```python
from build123d import *

# Parameters (mm, degrees)
SKETCH1_R           = 3.3782
SKETCH1_R_2         = 6
SKETCH1_R_3         = 8
BOSS_EXTRUDE1_DEPTH = 4.826
SKETCH2_W           = 4.826
SKETCH2_H           = 25.4
BOSS_EXTRUDE2_DEPTH = 4.826
SKETCH3_W           = 4.826
SKETCH3_H           = 25.4
CUT_EXTRUDE1_DEPTH  = 4.826
SKETCH4_W           = 4.826
SKETCH4_H           = 25.4
BOSS_EXTRUDE3_DEPTH = 4.826
SKETCH5_W           = 4.826
SKETCH5_H           = 25.4
CUT_EXTRUDE2_DEPTH  = 4.826
SKETCH6_W           = 4.826
SKETCH6_H           = 25.4
CUT_EXTRUDE3_DEPTH  = 9.652
SKETCH7_W           = 25.4
SKETCH7_H           = 4.826
CUT_EXTRUDE4_DEPTH  = 5.826
SKETCH9_W           = 4.826
SKETCH9_H           = 25.4
CUT_EXTRUDE5_DEPTH  = 5.826
BOSS_EXTRUDE4_DEPTH = 4.826
SKETCH11_R          = 4
CUT_EXTRUDE6_DEPTH  = 5.826


with BuildPart() as part:
    # Sketch1 → Boss-Extrude1 (new body)
    with BuildSketch(Plane.XY):
        with BuildLine():
            ThreePointArc((192.003501193, 390.374510077), (153.520537835, 394.589080012), (116.861974256, 407.032985542))
            Line((116.861974256, 407.032985542), (-86.189766395, 501.71756721))
            Line((-86.189766395, 501.71756721), (-86.189766395, 476.31756721))
            Line((-86.189766395, 476.31756721), (-81.363766395, 476.31756721))
            Line((-81.363766395, 476.31756721), (-81.363766395, 450.91756721))
            Line((-81.363766395, 450.91756721), (-86.189766395, 450.91756721))
            Line((-86.189766395, 450.91756721), (-86.189766395, 425.51756721))
            Line((-86.189766395, 425.51756721), (-81.363766395, 425.51756721))
            Line((-81.363766395, 425.51756721), (-81.363766395, 400.11756721))
            Line((-81.363766395, 400.11756721), (-86.189766395, 400.11756721))
            Line((-86.189766395, 400.11756721), (-86.189766395, 374.71756721))
            Line((-86.189766395, 374.71756721), (116.861974256, 280.032985542))
            ThreePointArc((116.861974256, 280.032985542), (153.520537835, 267.589080012), (192.003501193, 263.374510077))
            ThreePointArc((192.003501193, 263.374510077), (201.203503254, 261.71550325), (209.244538804, 256.947475478))
            ThreePointArc((209.244538804, 256.947475478), (225.871079853, 250.749510077), (242.497620902, 256.947475478))
            ThreePointArc((242.497620902, 256.947475478), (250.538656453, 261.71550325), (259.738658513, 263.374510077))
            Line((259.738658513, 263.374510077), (387.768126915, 263.374510077))
            ThreePointArc((387.768126915, 263.374510077), (401.20665362, 260.925821414), (412.917790929, 253.894510077))
            ThreePointArc((412.917790929, 253.894510077), (429.684233605, 247.574510077), (446.45067628, 253.894510077))
            ThreePointArc((446.45067628, 253.894510077), (458.161813589, 260.925821414), (471.600340294, 263.374510077))
            Line((471.600340294, 263.374510077), (624.413499087, 263.374510077))
            ThreePointArc((624.413499087, 263.374510077), (627.977205024, 263.123267502), (631.470410593, 262.374510077))
            ThreePointArc((631.470410593, 262.374510077), (645.584233605, 260.374510077), (659.698056616, 262.374510077))
            ThreePointArc((659.698056616, 262.374510077), (663.191262186, 263.123267502), (666.754968122, 263.374510077))
            Line((666.754968122, 263.374510077), (790.110233605, 263.374510077))
            Line((790.110233605, 263.374510077), (790.110233605, 288.774510077))
            Line((790.110233605, 288.774510077), (785.284233605, 288.774510077))
            Line((785.284233605, 288.774510077), (785.284233605, 314.174510077))
            Line((785.284233605, 314.174510077), (790.110233605, 314.174510077))
            Line((790.110233605, 314.174510077), (790.110233605, 339.574510077))
            Line((790.110233605, 339.574510077), (785.284233605, 339.574510077))
            Line((785.284233605, 339.574510077), (785.284233605, 364.974510077))
            Line((785.284233605, 364.974510077), (790.110233605, 364.974510077))
            Line((790.110233605, 364.974510077), (790.110233605, 390.374510077))
            Line((790.110233605, 390.374510077), (192.003501193, 390.374510077))
        make_face()
        with BuildLine():
            ThreePointArc((-26.914752452, 387.434325035), (-24.580466803, 381.020927923), (-30.993863915, 378.686642274))
            Line((-30.993863915, 378.686642274), (-65.524190601, 394.788398047))
            ThreePointArc((-65.524190601, 394.788398047), (-67.85847625, 401.201795158), (-61.445079138, 403.536080807))
            Line((-61.445079138, 403.536080807), (-26.914752452, 387.434325035))
        make_face(mode=Mode.SUBTRACT)
        with Locations((85.260233605, 377.674510077)):
            Circle(SKETCH1_R, mode=Mode.SUBTRACT)
        with Locations((-49.613766395, 425.51756721)):
            Circle(SKETCH1_R, mode=Mode.SUBTRACT)
        with Locations((225.871079853, 276.149510077)):
            Circle(SKETCH1_R_2, mode=Mode.SUBTRACT)
        with Locations((167.810233605, 295.124510077)):
            Circle(SKETCH1_R, mode=Mode.SUBTRACT)
        with Locations((91.610233605, 326.874510077)):
            Circle(SKETCH1_R, mode=Mode.SUBTRACT)
        with Locations((-9.032874317, 365.922075979)):
            Circle(SKETCH1_R_2, mode=Mode.SUBTRACT)
        with Locations((180.510233605, 358.624510077)):
            Circle(SKETCH1_R, mode=Mode.SUBTRACT)
        with Locations((429.684233605, 272.974510077)):
            Circle(SKETCH1_R_2, mode=Mode.SUBTRACT)
        with Locations((378.858833605, 282.424510077)):
            Circle(SKETCH1_R, mode=Mode.SUBTRACT)
        with Locations((531.258833605, 282.424510077)):
            Circle(SKETCH1_R, mode=Mode.SUBTRACT)
        with Locations((759.884233605, 288.774510077)):
            Circle(SKETCH1_R, mode=Mode.SUBTRACT)
        with Locations((404.258833605, 345.924510077)):
            Circle(SKETCH1_R, mode=Mode.SUBTRACT)
        with Locations((531.258833605, 345.924510077)):
            Circle(SKETCH1_R, mode=Mode.SUBTRACT)
        with Locations((645.584233605, 311.174510077)):
            Circle(SKETCH1_R_3, mode=Mode.SUBTRACT)
        with Locations((734.484233605, 352.274510077)):
            Circle(SKETCH1_R, mode=Mode.SUBTRACT)
    extrude(amount=BOSS_EXTRUDE1_DEPTH)

    # Sketch2 → Boss-Extrude2 (add)
    with BuildSketch(Plane(origin=(785.284233605, 0, 0), x_dir=(0, 0, -1), z_dir=(1, 0, 0))):
        with Locations((-2.413, 352.274510077)):
            Rectangle(SKETCH2_W, SKETCH2_H)
        with Locations((-2.413, 301.474510077)):
            Rectangle(SKETCH2_W, SKETCH2_H)
    extrude(amount=BOSS_EXTRUDE2_DEPTH)

    # Sketch3 → Cut-Extrude1 (cut)
    with BuildSketch(Plane(origin=(790.110233605, 0, 0), x_dir=(0, 0, -1), z_dir=(1, 0, 0))):
        with Locations((-2.413, 377.674510077)):
            Rectangle(SKETCH3_W, SKETCH3_H)
        with Locations((-2.413, 326.874510077)):
            Rectangle(SKETCH3_W, SKETCH3_H)
        with Locations((-2.413, 276.074510077)):
            Rectangle(SKETCH3_W, SKETCH3_H)
    extrude(amount=-CUT_EXTRUDE1_DEPTH, mode=Mode.SUBTRACT)

    # Sketch4 → Boss-Extrude3 (add)
    with BuildSketch(Plane.ZY.offset(81.363766395)):
        with Locations((2.413, 463.61756721)):
            Rectangle(SKETCH4_W, SKETCH4_H)
        with Locations((2.413, 412.81756721)):
            Rectangle(SKETCH4_W, SKETCH4_H)
    extrude(amount=BOSS_EXTRUDE3_DEPTH)

    # Sketch5 → Cut-Extrude2 (cut)
    with BuildSketch(Plane.ZY.offset(86.189766395)):
        with Locations((2.413, 387.41756721)):
            Rectangle(SKETCH5_W, SKETCH5_H)
        with Locations((2.413, 438.21756721)):
            Rectangle(SKETCH5_W, SKETCH5_H)
        with Locations((2.413, 489.01756721)):
            Rectangle(SKETCH5_W, SKETCH5_H)
    extrude(amount=-CUT_EXTRUDE2_DEPTH, mode=Mode.SUBTRACT)

    # Sketch6 → Cut-Extrude3 (cut)
    with BuildSketch(Plane(origin=(790.110233605, 0, 0), x_dir=(0, 0, -1), z_dir=(1, 0, 0))):
        with Locations((-2.413, 352.274510077)):
            Rectangle(SKETCH6_W, SKETCH6_H)
        with Locations((-2.413, 301.474510077)):
            Rectangle(SKETCH6_W, SKETCH6_H)
    extrude(amount=-CUT_EXTRUDE3_DEPTH, mode=Mode.SUBTRACT)

    # Sketch7 → Cut-Extrude4 (cut, through all)
    with BuildSketch(Plane.XY.offset(4.826)):
        with Locations((293.603501193, 387.961510077)):
            Rectangle(SKETCH7_W, SKETCH7_H)
        with Locations((344.403501193, 387.961510077)):
            Rectangle(SKETCH7_W, SKETCH7_H)
        with Locations((242.803501193, 387.961510077)):
            Rectangle(SKETCH7_W, SKETCH7_H)
    extrude(amount=-CUT_EXTRUDE4_DEPTH, mode=Mode.SUBTRACT)

    # Sketch9 → Cut-Extrude5 (cut, through all)
    with BuildSketch(Plane(origin=(0, 0, 0), x_dir=(-1, 0, 0), z_dir=(0, 0, -1))):
        with Locations((-354.690501193, 352.274510077)):
            Rectangle(SKETCH9_W, SKETCH9_H)
        with Locations((-354.690501193, 301.474510077)):
            Rectangle(SKETCH9_W, SKETCH9_H)
        with Locations((-232.516501193, 301.474510077)):
            Rectangle(SKETCH9_W, SKETCH9_H)
        with Locations((-232.516501193, 352.274510077)):
            Rectangle(SKETCH9_W, SKETCH9_H)
    extrude(amount=-CUT_EXTRUDE5_DEPTH, mode=Mode.SUBTRACT)

    # Sketch10 → Boss-Extrude4 (add)
    with BuildSketch(Plane.XY.offset(4.826)):
        with BuildLine():
            ThreePointArc((580.854886872, 263.374510077), (585.212430925, 261.14348344), (590.047133605, 260.374510077))
            Line((590.047133605, 260.374510077), (645.584233605, 260.374510077))
            ThreePointArc((645.584233605, 260.374510077), (638.456821732, 260.876995228), (631.470410593, 262.374510077))
            ThreePointArc((631.470410593, 262.374510077), (627.977205024, 263.123267502), (624.413499087, 263.374510077))
            Line((624.413499087, 263.374510077), (580.854886872, 263.374510077))
        make_face()
        with BuildLine():
            ThreePointArc((659.698056616, 262.374510077), (652.711645477, 260.876995228), (645.584233605, 260.374510077))
            Line((645.584233605, 260.374510077), (701.172133605, 260.374510077))
            ThreePointArc((701.172133605, 260.374510077), (706.006836284, 261.14348344), (710.364380338, 263.374510077))
            Line((710.364380338, 263.374510077), (666.754968122, 263.374510077))
            ThreePointArc((666.754968122, 263.374510077), (663.191262186, 263.123267502), (659.698056616, 262.374510077))
        make_face()
    extrude(amount=-BOSS_EXTRUDE4_DEPTH)

    # Sketch11 → Cut-Extrude6 (cut, through all)
    with BuildSketch(Plane.XY.offset(4.826)):
        with Locations((590.047133605, 387.082410077)):
            Circle(SKETCH11_R)
        with Locations((701.172133605, 387.082410077)):
            Circle(SKETCH11_R)
        with Locations((701.172133605, 275.957410077)):
            Circle(SKETCH11_R)
        with Locations((590.047133605, 240.977875999)):
            Circle(SKETCH11_R)
    extrude(amount=-CUT_EXTRUDE6_DEPTH, mode=Mode.SUBTRACT)


solid = part.part
```
The model under review builds one solid part; all positions refer to its coordinate system, in mm. A direction names the side the tool comes from. Round coordinates to 2 decimals unless told otherwise and drop trailing zeros. Write each loop counter-clockwise with the first axis right and the second up, starting at its lowest first coordinate (ties: lowest second). Pieces come first, ordered by that corner, then holes. Notation, with made-up numbers: (3, 35.5) - (24, 35.5) arc R17 ccw to (24, 62.5) - close; hole circle Ø6 at (85.25, -13). An arc over 180 degrees is marked (long way). One line per question, with ' | ' between items.
Item 1: To check wall thickness, follow probe 1 along Y at (x, z) = (352.5, 1.15); probe 2 along Y at (x, z) = (325.5, 4.2); probe 3 along X at (y, z) = (377.5, 1.6). State the ranges of each line that lie inside material, in increasing order.
Resolved:
probe 1: y = 263.37 to 288.77, 314.17 to 339.57, 364.97 to 385.55 | probe 2: y = 263.37 to 390.37 | probe 3: x = -81.36 to 81.89, 88.63 to 785.28
Item 2: The part is to be moulded in two halves that separate along Y. For faces 1 (the face through (639.236, 306.307, 2.379)), 2 (the face through (343, 347, 4.826)), 3 (the face through (154.051, 394.472, 2.379)), say which applies: pulls with the +Y half, pulls with the -Y half, needs draft (parallel to the pull), parting line crosses it, or undercut.
Resolved:
face 1: undercut | face 2: needs draft | face 3: pulls with the +Y half
Item 3: For faces 4 (the face through (19.14, 452.6, 2.38)), 5 (the face through (-44.422, 395.598, 2.379)), list the 3-axis set-ups (+Z, -Z, +X, -X, +Y, -Y) from which the entire face can be reached by the end or side of a thin tool; tool diameter is ignored.
Resolved:
face 4: +Z, -Z, +X, +Y | face 5: +Z, -Z
Item 4: For P1, Ø5.5, axis at x = 167.81, y = 295.12, coming from the +Z side; P2, Ø2, axis at y = 468.5, z = 1.5, coming from the +X side; P3, Ø2.5, axis at x = -83, z = 1.5, coming from the -Y side; P4, Ø1.5, axis at y = 331.5, z = 0.5, coming from the -X side, all flat-tipped, find the tip position at first contact; note any pin that passes through.
Resolved:
P1: passes through | P2: stops at x = -12.81 | P3: stops at y = 372.65 | P4: stops at x = 4.88
Item 5: Add section B-B, the plane z = 3.75. State how many separate pieces and enclosed holes the cut face has, then the cut area to 3 significant figures.
Resolved:
separate pieces: 1 | enclosed holes: 21 | area: 109,000 mm2
Item 6: Add section A-A, the plane x = 513.5. Give the boundary of the cut face in (y, z).
Resolved:
outline: (263.37, 0) - (390.37, 0) - (390.37, 4.83) - (263.37, 4.83) - close
